Autodesk Inventor part; units mm, degrees
ref_plane "Work Plane1" through (32.7477, 110, 0) normal (0, 0.7071, -0.7071) x (-1, 0, 0)
ref_plane "YZ Plane" through (0, 0, 0) normal (1, 0, 0) x (0, 1, 0)
ref_plane "XZ Plane" through (0, 0, 0) normal (0, 1, 0) x (-1, 0, 0)
sketch "Sketch1" plane through (0, 0, 0) normal (0, 1, 0) x (-1, 0, 0)
  circle A0 centre (0, 0) radius 68
  circle A1 centre (0, 0) radius 70
  dimension "d0" = 2
  dimension "d1" = 140
extrude "Extrusion1" add sketch "Sketch1" along normal blind 180
sketch "Sketch2" plane through (0, 0, 0) normal (0, 0, 1) x (1, 0, 0)
  line L0 (-58, 20) -> (58, 20)
  line L1 (58, 20) -> (58, 62)
  line L2 (58, 62) -> (-58, 62)
  line L3 (-58, 62) -> (-58, 20)
  line L4 (70, 0) -> (-70, 0)
  point P0 (0, 0)
  point P1 (0, 0)
  dimension "d4" = 42
  dimension "d5" = 116
  dimension "d6" = 20
  dimension "d7" = 58
extrude "Extrusion2" cut sketch "Sketch2" against normal through all
sketch "Sketch3" plane through (0, 0, 0) normal (0, 0, 1) x (1, 0, 0)
  line L0 (32.7477, 110) -> (-36.5, 110)
  line L1 (70, 0) -> (-70, 0)
  point P0 (0, 0)
  point P1 (-1.8762, 110)
  dimension "d12" = 110
ref_plane "Work Plane1" through (32.7477, 110, 0) normal (0, 0.7071, -0.7071) x (-1, 0, 0)
sketch "Sketch4" plane through (32.7477, 110, 0) normal (0, 0.7071, -0.7071) x (-1, 0, 0)
  circle A0 centre (32.7477, -40) radius 35
  line L0 (0, 0) -> (69.2476, 0)
  point P0 (32.7477, -77.7817)
  point P1 (34.6238, 0)
  point P2 (34.6238, 0)
  dimension "d11" = 70
  dimension "d15" = 40
extrude "Extrusion3" cut sketch "Sketch4" along normal through all
properties part number "Outer shaft"
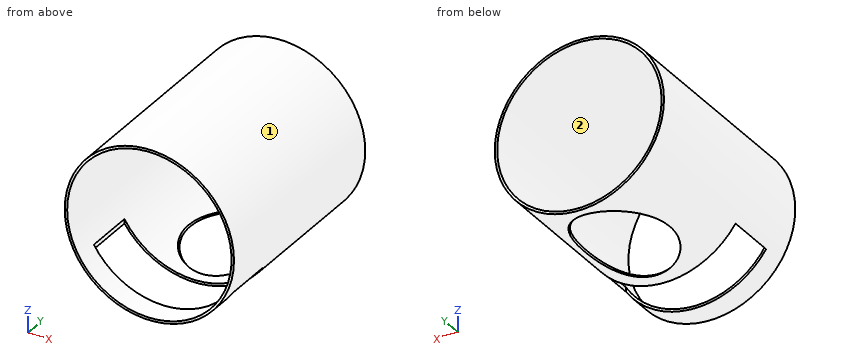
The listing builds one solid part. Answer for the finished solid, in the listing's coordinates (mm). Face numbers are marked on the shaded views. Give positions to 0.01 mm unless a question says otherwise; leave off trailing zeros. Order: outer loops, then holes, each group sorted by start corner. A loop starts at its lowest first (then second) coordinate and runs counter-clockwise, first axis right, second up. Notation, with made-up numbers: (15, 77.25) - (52, 77.25) arc R18 ccw to (52, 86.25) - close; hole circle Ø2 at (64.5, 71.25). An arc over 180 degrees is marked (long way). Use one line per item in the form item = value.
1) Consider probe 1 along Z at (x, y) = (0, 109); probe 2 along X at (y, z) = (55, 6.5); probe 3 along X at (y, z) = (125, 14.5). Determine where each line is inside the solid, lowest interval first. Write a range as [from, to].
Verdict:
probe_1 = [68, 70]
probe_2 = [-69.7, -67.69], [67.69, 69.7]
probe_3 = [-68.48, -66.44], [66.44, 68.48]
2) Find section B-B on x = 38. Determine the outline of the cut face in (y, z), and give its area (3 significant figures).
Verdict:
outline = (0, -58.79) - (20, -58.79) - (20, -56.39) - (0, -56.39) - close; (0, 56.39) - (180, 56.39) - (180, 58.79) - (0, 58.79) - close; (62, -58.79) - (180, -58.79) - (180, -56.39) - (62, -56.39) - close
area = 762 mm^2
3) Find section A-A on z = 0. Determine the outline of the cut face in (x, y).
Verdict:
outline = (-70, 0) - (-68, 0) - (-68, 180) - (-70, 180) - close; (68, 0) - (70, 0) - (70, 180) - (68, 180) - close
4) Find section C-C on x = 0. Determine the outline of the cut face in (y, z).
Verdict:
outline = (0, -70) - (20, -70) - (20, -68) - (0, -68) - close; (0, 68) - (180, 68) - (180, 70) - (0, 70) - close; (62, -70) - (73.93, -70) - (71.93, -68) - (62, -68) - close; (170.93, -68) - (172.93, -70) - (180, -70) - (180, -68) - close
5) The mould has two halves that part along Z. Classify the marked faces 1 and 2: released by +Z, released by -Z, zero draft, split by the parting line, or undercut.
Verdict:
face_1 = split by the parting line
face_2 = undercut
6) Each of these flat-tipped pins is pushed along its axis until it touches: pin 1 (5 mm diameter, centred on y = 149, z = -48.5, fed in from +X); pin 2 (6 mm diameter, centred on y = 125, z = -32, fed in from +X); pin 3 (6 mm diameter, centred on y = 79, z = 50, fed in from -X); pin 4 (17.5 mm diameter, centred on x = -1, z = -54, fed in from -Y). Where does it stop, or does it pass through?
Verdict:
pin_1 = 52.76
pin_2 = 63.71
pin_3 = -51.87
pin_4 = through
7) Find section D-D on z = -48. Determine the outline of the cut face in (x, y), and give its area (3 significant figures).
Verdict:
outline = (-50.95, 0) - (-48.17, 0) - (-48.17, 20) - (-50.95, 20) - close; (-50.95, 62) - (-48.17, 62) - (-48.17, 180) - (-50.95, 180) - close; (48.17, 0) - (50.95, 0) - (50.95, 20) - (48.17, 20) - close; (48.17, 62) - (50.95, 62) - (50.95, 180) - (48.17, 180) - close
area = 769 mm^2
